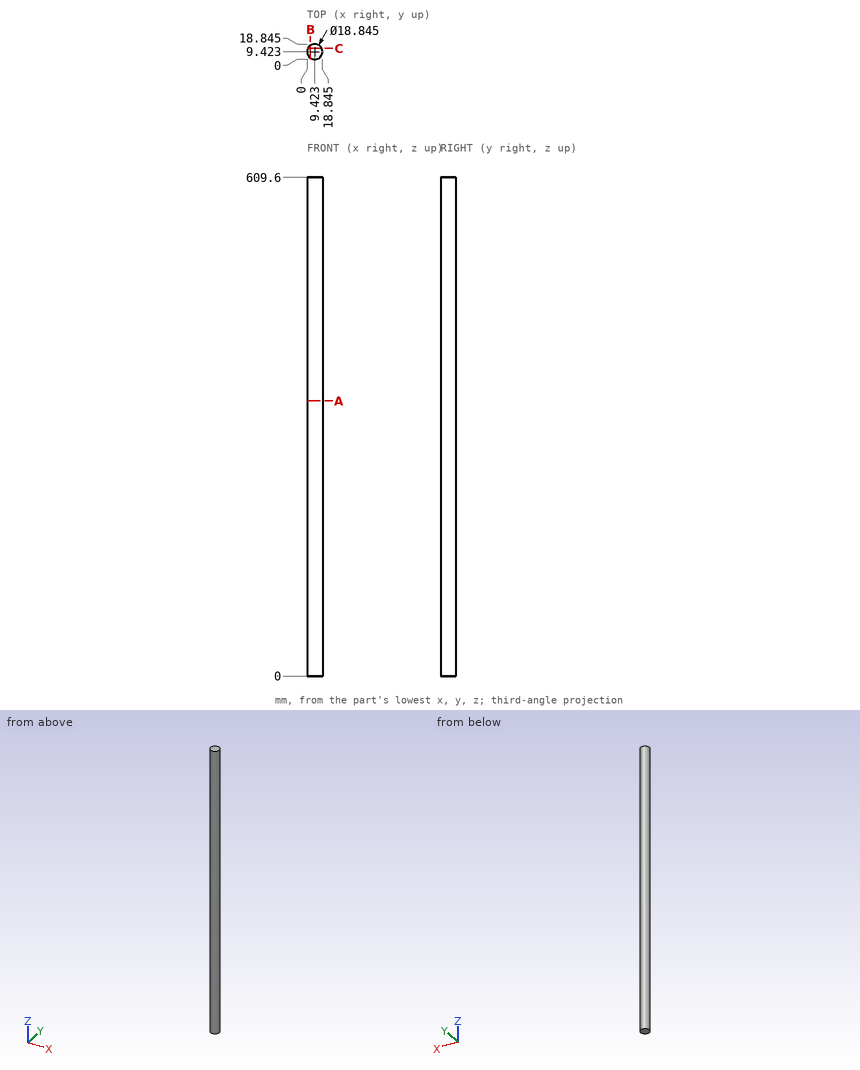
Study the drawing (mm; zero at the part's minimum x, y, z) and answer. Give positions to 0.01 mm unless a question says otherwise; leave off trailing zeros. Order: outer loops, then holes, each group sorted by start corner. A loop starts at its lowest first (then second) coordinate and runs counter-clockwise, first axis right, second up. Notation, with made-up numbers: (65.5, 76) -> (116.5, 76) arc R17 ccw to (116.5, 90) -> close; hole circle Ø11 at (-29.75, 59). An arc over 180 degrees is marked (long way). Write item = value, one per line.
1. Given pin 1 (6 mm diameter, centred on y = 13, z = 448, fed in from +X); pin 2 (4 mm diameter, centred on y = 16.5, z = 428.5, fed in from -X) (1 decimal); pin 3 (1 mm diameter, centred on x = 12.5, z = 399.5, fed in from +Y), each flat-ended and moving along its own axis, determine where each tip first touches the part or whether it passes through.
Numbers:
pin_1 = 18.83
pin_2 = 1.5
pin_3 = 18.49
2. A cutting plane is placed at C-C, the plane y = 13.5. Write down the section's boundary in (x, z).
Numbers:
outline = (0.93, 0) -> (17.92, 0) -> (17.92, 609.6) -> (0.93, 609.6) -> close
3. A cutting plane is placed at A-A, the plane z = 336.5. Write down the section's boundary in (x, y) (1 decimal), and give its area (3 significant figures).
Numbers:
outline = circle Ø18.8 at (9.4, 9.4)
area = 279 mm²
4. A cutting plane is placed at B-B, the plane x = 4. Write down the section's boundary in (y, z).
Numbers:
outline = (1.72, 0) -> (17.13, 0) -> (17.13, 609.6) -> (1.72, 609.6) -> close
5. Straight lines are drawn through the part: line 1 along Y through (x, z) = (9, 58); line 2 along X through (y, z) = (8.5, 342) (1 decimal); line 3 along X through (y, z) = (16.5, 362) (1 decimal). For each, find the intervals that lie inside material, in ascending order.
Numbers:
line_1 = 0.01 to 18.84
line_2 = 0 to 18.8
line_3 = 3.2 to 15.6
